Check sheet for the modelled part. Datum: model origin and axes. Units: mm. Face numbers are marked on the shaded views. A direction names the side the tool comes from. Coordinates: 2 decimals unless noted, no trailing zeros. Write each loop counter-clockwise with the first axis right and the second up, starting at its lowest first coordinate (ties: lowest second). Pieces come first, ordered by that corner, then holes. Notation, with made-up numbers: (-11.5, 67.25) - (1.5, 67.25) arc R14 cw to (1.5, 72.25) - close; hole circle Ø4 at (88.25, -28.5). An arc over 180 degrees is marked (long way). Write each question's results on one line, items separated by ' | '.
from build123d import *

# Parameters (mm, degrees)
F6_R      = 5.225
F7_DEPTH  = 1
F5_R      = 4.225
F5_R_2    = 3.225
F8_DEPTH  = 4.3
F9_R      = 3.225
F9_R_2    = 2.75
F10_DEPTH = 0.95
F11_SIZE  = 0.47499
F12_SIZE  = 0.475


# Not quite as in the source:
# - a fillet or chamfer is up to 0.001 mm smaller than in the source, because OpenCascade refuses the exact size


with BuildPart() as f7:
    # F6 (on face) → F7 (new body)
    with BuildSketch(Plane.XY):
        Circle(F6_R)
    extrude(amount=-F7_DEPTH)



with BuildPart() as f7b:
    # F5 (on Top) → F7, piece 2 (new body)
    with BuildSketch(Plane.XY):
        Circle(F5_R)
        Circle(F5_R_2, mode=Mode.SUBTRACT)
    extrude(amount=-F7_DEPTH)


with BuildPart() as f7_1:
    add(f7.part)

    add(f7b.part)  # F8 merges F7b
    # F5 (on Top) → F8 (join)
    with BuildSketch(Plane.XY):
        Circle(F5_R)
        Circle(F5_R_2, mode=Mode.SUBTRACT)
    extrude(amount=F8_DEPTH)

    # F9 (on face) → F10 (join)
    with BuildSketch(Plane.XY.offset(4.3)):
        Circle(F9_R)
        Circle(F9_R_2, mode=Mode.SUBTRACT)
    extrude(amount=-F10_DEPTH)

    # F11 (size 0.475 in the source; OpenCascade refuses exactly that, so slightly less here)
    f11_edges = [f7_1.edges().sort_by_distance(p)[0] for p in [
        (-2.75, 0, 3.35),
    ]]
    chamfer(f11_edges, length=F11_SIZE)

    # F12
    f12_edges = [f7_1.edges().sort_by_distance(p)[0] for p in [
        (-3.225, 0, 0),
    ]]
    chamfer(f12_edges, length=F12_SIZE)


solid = f7_1.part
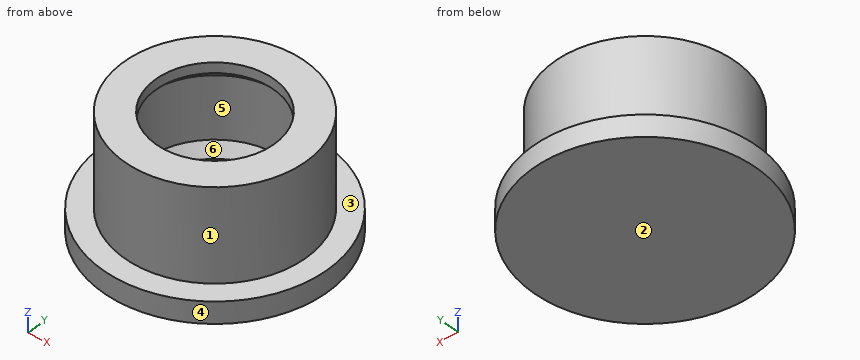
1. Sectioned sample at B-B (z = 1). Record the cut outline in (x, y) (3 decimals), then the cut area to 3 significant figures.
Values follow:
outline: circle Ø8.45 at (0, 0); hole circle Ø6.45 at (0, 0) | area: 23.4 mm^2
2. Go/stop test with flat-tipped pins: pin 1 (5 mm diameter, centred on x = -2, y = -0.5, fed in from +Z); pin 2 (3 mm diameter, centred on x = -0.5, y = 0.5, fed in from +Z). Record where each tip stops, or that it passes through.
Values follow:
pin 1: stops at z = 4.3 | pin 2: stops at z = 0
3. Draft check along Y on the marked faces 3, 4, 5 and 6. Enter one of: pulls with the +Y half, pulls with the -Y half, needs draft (parallel to the pull), parting line crosses it, or undercut.
Values follow:
face 3: needs draft | face 4: parting line crosses it | face 5: undercut | face 6: undercut
4. Sectioned sample at D-D (z = -0.55). Record the cut outline in (x, y) (3 decimals).
Values follow:
outline: circle Ø10.45 at (0, 0)
5. Material ranges on L1, parallel to Y at x = 0, z = 2.25 (3 decimals); L2, parallel to Y at x = 0, z = 4.1 (3 decimals); L3, parallel to X at y = -0.5, z = 0.6, recorded low to high. Write a range as [from, to].
Values follow:
L1: y = [-4.225, -3.225], [3.225, 4.225] | L2: y = [-4.225, -2.75], [2.75, 4.225] | L3: x = [-4.2, -3.19], [3.19, 4.2]
6. Access from +Z, -Z, +X, -X, +Y, -Y to the whole of each face (thin tool, end or side, straight path). Record for the marked faces 1 and 2.
Values follow:
face 1: +Z | face 2: -Z, +X, -X, +Y, -Y
